Autodesk Inventor part; units mm, degrees
ref_plane "YZ Plane" through (0, 0, 0) normal (1, 0, 0) x (0, 1, 0)
ref_plane "XZ Plane" through (0, 0, 0) normal (0, 1, 0) x (-1, 0, 0)
ref_plane "XY Plane" through (0, 0, 0) normal (0, 0, 1) x (1, 0, 0)
sketch "Boceto1" plane through (0, 0, 0) normal (0, 1, 0) x (-1, 0, 0)
  circle A0 centre (0, 0) radius 79
  circle A1 centre (0, 0) radius 12
  dimension "d0" = 158
  dimension "d1" = 24
extrude "Extrusión1" add sketch "Boceto1" along normal blind 27
chamfer "Chaflán1" distance 3 angle 45 1 edges at (79, 27, 0) measured on face at (-12.739, 27, -55.0245)
sketch "Boceto2" plane through (0, 27, 0) normal (0, 1, 0) x (1, 0, 0)
  circle A0 centre (0, 0) radius 64 construction
  line L0 (0, 0) -> (64, 0) construction
  point P0 (32, 55.4256)
  point P1 (-32, 55.4256)
  point P2 (-64, 0)
  point P3 (-32, -55.4256)
  point P4 (32, -55.4256)
  dimension "d7" = 128
  dimension "d10" = 360
hole "Agujero1" at (64, 27, 0) at (32, 27, -55.4256) at (-32, 27, -55.4256) at (-64, 27, 0) at (-32, 27, 55.4256) at (32, 27, 55.4256) direction (0, -1, 0) diameter 12.5 end through all counterbore diameter 19.25 counterbore depth 12.5
sketch "Boceto3" plane through (0, 27, 0) normal (0, 1, 0) x (1, 0, 0)
  line L0 (0, 0) -> (34, 0) construction
  dimension "d19" = 34
hole "Agujero2" at (34, 27, 0) direction (0, -1, 0) diameter 14 depth 17
sketch "Boceto5" plane through (0, 0, 0) normal (0, 0, 1) x (1, 0, 0)
  line L0 (79, 0) -> (-79, 0) construction
  line L1 (79, 0) -> (33, 0) construction
  line L2 (33, 0) -> (44, 0)
  line L3 (44, 0) -> (44, 6)
  line L4 (44, 6) -> (33, 6)
  line L5 (33, 6) -> (33, 0)
  line L6 (0, 0) -> (0, 42.6021) construction
  dimension "d29" = 46
  dimension "d30" = 11
  dimension "d31" = 6
  dimension "d32" = 11
revolve "Revolución1" cut sketch "Boceto5" angle 360 about axis through (0, 0, 0) along (0, 1, 0)
properties part number "2_VálvulaSuperior"
Could you check a few things on this model? Use its own coordinates, in mm. A direction names the side the tool comes from. Coordinates: 2 decimals unless noted, no trailing zeros. Order: outer loops, then holes, each group sorted by start corner. A loop starts at its lowest first (then second) coordinate and runs counter-clockwise, first axis right, second up. Notation, with made-up numbers: M -30,71 L -26,71 A11 cw -26,90 Z; hole C 67,-17 d3. An arc over 180 degrees is marked long. Use a Markdown table: item, result. Add a question column.
Q1. I want a section at A-A on x = 0. List the corners of the cut face in (y, z) for me.
Q2. We'd pull the mould along X, two halves only. Please class faces 1 (the cylindrical face through (40.539, 20.662, 59.867)), 2 (the cylindrical face through (58.23, 11.83, -53.39)), 3 (the cylindrical face through (11.99, 13.31, -0.53)), 4 (the flat face through (-16, 27, 1)): pulls with the +X half, pulls with the -X half, needs draft (parallel to the pull), parting line crosses it, or undercut.
Q3. If I drill on L1, parallel to Z at x = 32, y = 19.5; L2, parallel to Z at x = 0, y = 16; L3, parallel to X at y = 18.5, z = 57, over which ranges is the centre line in solid material (lowest first)?
Q4. Which directions (+Z, -Z, +X, -X, +Y, -Y) give clear straight access to the entire face, cutting with the end or side of a thin tool? Please do faces 5 (the cylindrical face through (-26.14, 20.66, -63.06)), 6 (the flat face through (-34, 0, -34)), 7 (the flat face through (6, 6, -33)).
Q5. I want a section at B-B on y = 12.5. Give the number of separate pieces and of enclosed holes in the cut face, then the cut area to 3 significant figures.
Q6. I'm going to push flat-ended pins straight in: pin 1 (21 mm diameter, centred on x = -32.5, z = 52, fed in from +Y); pin 2 (12 mm diameter, centred on y = 8, z = -11, fed in from -X); pin 3 (6 mm diameter, centred on x = 66.5, z = 4.5, fed in from +Y); pin 4 (3 mm diameter, centred on x = 8.5, y = 10, fed in from -Z). Where does each tip first touch, or does it pass through?
Checked values:
| question | item | result |
|---|---|---|
| 1 | outline | M 0,-79 L 24,-79 L 27,-76 L 27,-12 L 0,-12 L 0,-33 L 6,-33 L 6,-44 L 0,-44 Z; M 0,12 L 27,12 L 27,76 L 24,79 L 0,79 L 0,44 L 6,44 L 6,33 L 0,33 Z |
| 2 | face 1 | undercut |
| 2 | face 2 | parting line crosses it |
| 2 | face 3 | undercut |
| 2 | face 4 | needs draft |
| 3 | L1 | -72.23 to -65.05, -45.8 to -6.71, 6.71 to 45.8, 65.05 to 72.23 |
| 3 | L2 | -79 to -12, 12 to 79 |
| 3 | L3 | -54.7 to -41.5, -22.5 to 22.5, 41.5 to 54.7 |
| 4 | face 5 | +Y |
| 4 | face 6 | +Z, -Z, +X, -X, -Y |
| 4 | face 7 | -Y |
| 5 | separate pieces | 1 |
| 5 | enclosed holes | 8 |
| 5 | area | 18,300 mm² |
| 6 | pin 1 | y = 27 |
| 6 | pin 2 | x = -78.84 |
| 6 | pin 3 | y = 14.5 |
| 6 | pin 4 | z = -78.69 |
